Read the model definition and answer for the solid it produces. Units are mm, in the model's axes. Face numbers are marked on the shaded views. A direction names the side the tool comes from. Coordinates: 2 decimals unless noted, no trailing zeros. Write each loop counter-clockwise with the first axis right and the second up, starting at its lowest first coordinate (ties: lowest second). Pieces come first, ordered by that corner, then holes. Notation, with made-up numbers: (-23.75, 16.5) -> (-18.75, 16.5) arc R23 ccw to (-18.75, 30.5) -> close; hole circle Ø8 at (17, 6). An arc over 180 degrees is marked (long way). Write item = value, one per line. Start each with the question number.
1) Section A-A (y = 3) is taken. Determine the outline of the cut face in (x, z), plus the area to 3 significant figures.
2) For a pull along Y with two mould halves and no side action, classify the marked faces 5, 6 and 7 as released by +Y, released by -Y, zero draft, split by the parting line, or undercut.
3) A tool of negligible diameter and unlimited length cuts with its end or side. For the marked faces 1, 2, 3 and 4, from which of +Z, -Z, +X, -X, +Y, -Y can it reach the whole face along a straight path? Write none if from no direction.
4) Section C-C (z = 42) is taken. Determine the outline of the cut face in (x, y).
5) Find the intervals of material crossed by line 1 along Y through (x, z) = (-46, 4.5); line 2 along Z through (x, y) = (-37, -27.5), in increasing order. Write a range as from..to.
6) Flat-ended cylindrical pins translate along their axes: pin 1 Ø7 at (x, z) = (-30, 4) entering from -Y; pin 2 Ø1 at (x, y) = (-15, -1.5) entering from -Z; pin 3 Ø8.5 at (x, y) = (-16.5, -15.5) entering from +Z; pin 4 Ø12 at (x, z) = (-32.5, 27.5) entering from -Y. Find the tip coordinate at first contact, or state that the pin passes through.
7) Section D-D (x = -22) is taken. Determine the outline of the cut face in (y, z), plus the area to 3 significant figures.
8) Section B-B (x = -33) is taken. Determine the outline of the cut face in (y, z), plus the area to 3 significant figures.
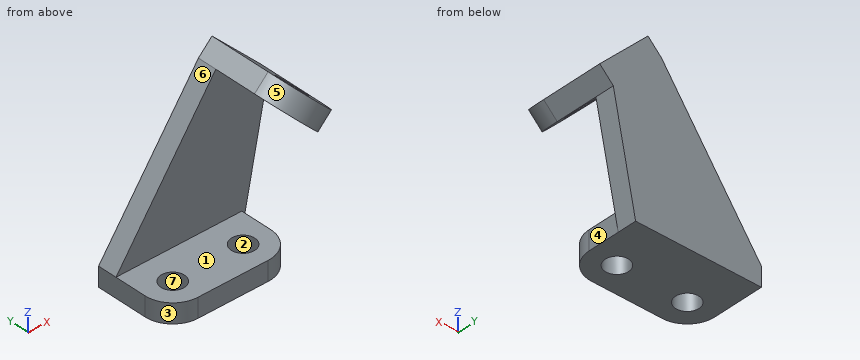
from build123d import *

# Parameters (mm, degrees)
F0_R     = 5.5
F1_DEPTH = 9
F3_DEPTH = 9
F4_R     = 7
F5_DEPTH = 9


with BuildPart() as f1:
    # F0 (on Top) → F1 (new body)
    with BuildSketch(Plane.XY):
        with BuildLine():
            Line((0, -15), (0, 0))
            Line((0, 0), (-59, 0))
            Line((-59, 0), (-59, -15))
            ThreePointArc((-59, -15), (-55.192388, -24.192388), (-46, -28))
            Line((-46, -28), (-13, -28))
            ThreePointArc((-13, -28), (-3.807612, -24.192388), (0, -15))
        make_face()
        with Locations((-46, -15)):
            Circle(F0_R, mode=Mode.SUBTRACT)
        with Locations((-13, -15)):
            Circle(F0_R, mode=Mode.SUBTRACT)
    extrude(amount=F1_DEPTH)

    # F2 (on face) → F3 (join)
    with BuildSketch(Plane(origin=(0, 0, 0), x_dir=(-1, 0, 0), z_dir=(0, 1, 0))):
        Polygon((59, 0), (59, 9), (12.163848, 75.313708), (-10.463569, 52.686292), (0, 0), align=None)
    extrude(amount=F3_DEPTH)

    # F4 (on face) → F5 (join)
    with BuildSketch(Plane(origin=(31.57493, 0, 31.57493), x_dir=(0.707107, 0, -0.707107), z_dir=(0.707107, 0, 0.707107))):
        with BuildLine():
            Line((-29.855973, 9), (-61.855973, 9))
            Line((-61.855973, 9), (-61.855973, -20))
            ThreePointArc((-61.855973, -20), (-45.855973, -36), (-29.855973, -20))
            Line((-29.855973, -20), (-29.855973, 9))
        make_face()
        with Locations((-45.855973, -20)):
            Circle(F4_R, mode=Mode.SUBTRACT)
    extrude(amount=F5_DEPTH)


solid = f1.part
Answer key:
q1.outline = (-59, 0) -> (0, 0) -> (10.46, 52.69) -> (16.83, 59.05) -> (-5.8, 81.68) -> (-12.16, 75.31) -> (-59, 9) -> close
q1.area = 3,430 mm^2
q2.face_5 = released by -Y
q2.face_6 = zero draft
q2.face_7 = undercut
q3.face_1 = +X, -X, -Y
q3.face_2 = -Z
q3.face_3 = +Z, -Z, -X, -Y
q3.face_4 = -Z, +X, -Y
q4.outline = (-35.69, 0) -> (8.34, 0) -> (8.34, 9) -> (-35.69, 9) -> close
q5.line_1 = -28..-20.5, -9.5..9
q5.line_2 = 0..9
q6.pin_1 = -28
q6.pin_2 = 0
q6.pin_3 = 9
q6.pin_4 = 0
q7.outline = (-28, 0) -> (9, 0) -> (9, 61.39) -> (0, 61.39) -> (0, 9) -> (-28, 9) -> close
q7.area = 804 mm^2
q8.outline = (-28, 0) -> (9, 0) -> (9, 45.81) -> (0, 45.81) -> (0, 9) -> (-28, 9) -> close
q8.area = 664 mm^2
